```python
from build123d import *

# Parameters (mm, degrees)
SKETCH_1_W               = 124
SKETCH_1_H               = 43
EXTRUDE_1_DEPTH          = 1.2
CUT_EXTRUDE_1_REACH      = 110.402
SKETCH_3_W               = 7.4
SKETCH_3_H               = 4.6
SKETCH_3_W_2             = 4.6
CUT_EXTRUDE_2_DEPTH      = 0.4
FILLET_1_R               = 3
EXTRUDE_START            = 5
EXTRUDE_5_DEPTH          = 5
SKETCH_7_W               = 0.8
SKETCH_7_H               = 5.4
EXTRUDE_6_DEPTH          = 33.335489
SKETCH_8_W               = 4.5
SKETCH_8_H               = 0.8
CUT_EXTRUDE_3_DEPTH      = 5
CHAMFER_2_SIZE           = 0.5
CUT_EXTRUDE_5_DEPTH      = 109.510329697
CUT_EXTRUDE_5_DEPTH_BACK = 109.510329697
FILLET_2_R               = 3
FILLET_3_R               = 1
FILLET_4_R               = 0.5
SKETCH_10_W              = 10
SKETCH_10_H              = 0.8
CUT_EXTRUDE_6_DEPTH      = 5


with BuildPart() as part:
    # Эскиз1 → Бобышка-Вытянуть1 (new body)
    with BuildSketch(Plane(origin=(0, 0, 0), x_dir=(1, 0, 0), z_dir=(0, 1, 0))):
        with Locations((43.92682215, 1.5)):
            Rectangle(SKETCH_1_W, SKETCH_1_H)
    extrude(amount=EXTRUDE_1_DEPTH)

    # Эскиз3 → Вырез-Вытянуть1 (cut, up to next)
    with BuildSketch(Plane.XZ, mode=Mode.PRIVATE) as cut_extrude_1_sk1:
        with Locations((-7.87317785, -0.05)):
            Rectangle(SKETCH_3_W, SKETCH_3_H)
    cut_extrude_1_tool1 = extrude(cut_extrude_1_sk1.sketch, amount=-CUT_EXTRUDE_1_REACH, mode=Mode.PRIVATE) & part.part
    # Эскиз3 → Вырез-Вытянуть1 (cut, up to next)
    with BuildSketch(Plane.XZ, mode=Mode.PRIVATE) as cut_extrude_1_sk2:
        with Locations((-7.57317785, -7.75)):
            Rectangle(SKETCH_3_W_2, SKETCH_3_H)
    cut_extrude_1_tool2 = extrude(cut_extrude_1_sk2.sketch, amount=-CUT_EXTRUDE_1_REACH, mode=Mode.PRIVATE) & part.part
    add(cut_extrude_1_tool1.solids().sort_by_distance((-7.873178, 0, -0.05))[0], mode=Mode.SUBTRACT)
    add(cut_extrude_1_tool2.solids().sort_by_distance((-7.573178, 0, -7.75))[0], mode=Mode.SUBTRACT)

    # Эскиз4 → Вырез-Вытянуть2 (cut)
    with BuildSketch(Plane(origin=(0, 1.2, 0), x_dir=(1, 0, 0), z_dir=(0, 1, 0))):
        with BuildLine():
            Line((4.110011464, 20.25), (7.343632837, 20.25))
            Line((7.343632837, 20.25), (29.42682215, 20.25))
            Line((29.42682215, 20.25), (29.42682215, -13.75))
            ThreePointArc((29.42682215, -13.75), (28.401695885, -16.224873734), (25.92682215, -17.25))
            Line((25.92682215, -17.25), (-13.07317785, -17.25))
            ThreePointArc((-13.07317785, -17.25), (-15.548051584, -16.224873734), (-16.57317785, -13.75))
            Line((-16.57317785, -13.75), (-16.57317785, 16.75))
            ThreePointArc((-16.57317785, 16.75), (-15.548051584, 19.224873734), (-13.07317785, 20.25))
            Line((-13.07317785, 20.25), (4.110011464, 20.25))
        make_face()
    extrude(amount=-CUT_EXTRUDE_2_DEPTH, mode=Mode.SUBTRACT)

    # Скругление1
    fillet_1_edges = [part.edges().sort_by_distance(p)[0] for p in [
        (-18.07317785, 0.6, -23),
        (105.92682215, 0.6, -23),
        (105.92682215, 0.6, 20),
        (-18.07317785, 0.6, 20),
    ]]
    fillet(fillet_1_edges, radius=FILLET_1_R)

    # Эскиз5 → Бобышка-Вытянуть5 (add)
    with BuildSketch(Plane(origin=(0, 1.2, 0), x_dir=(1, 0, 0), z_dir=(0, 1, 0)).offset(EXTRUDE_START)):
        with BuildLine():
            ThreePointArc((102.92682215, -19), (104.341035713, -18.414213562), (104.92682215, -17))
            Line((104.92682215, -17), (104.92682215, 20))
            ThreePointArc((104.92682215, 20), (104.341035713, 21.414213562), (102.92682215, 22))
            Line((102.92682215, 22), (-15.07317785, 22))
            ThreePointArc((-15.07317785, 22), (-16.487391412, 21.414213562), (-17.07317785, 20))
            Line((-17.07317785, 20), (-17.07317785, -17))
            ThreePointArc((-17.07317785, -17), (-16.487391412, -18.414213562), (-15.07317785, -19))
            Line((-15.07317785, -19), (102.92682215, -19))
        make_face()
        with BuildLine():
            Line((102.92682215, -18.2), (-15.07317785, -18.2))
            ThreePointArc((-15.07317785, -18.2), (-15.921705987, -17.848528137), (-16.27317785, -17))
            Line((-16.27317785, -17), (-16.27317785, -15.167744688))
            ThreePointArc((-16.27317785, -15.167744688), (-16.497356583, -14.474568837), (-16.57317785, -13.75))
            Line((-16.57317785, -13.75), (-16.57317785, 16.75))
            ThreePointArc((-16.57317785, 16.75), (-16.497356583, 17.474568837), (-16.27317785, 18.167744688))
            Line((-16.27317785, 18.167744688), (-16.27317785, 20))
            ThreePointArc((-16.27317785, 20), (-15.921705987, 20.848528137), (-15.07317785, 21.2))
            Line((-15.07317785, 21.2), (102.92682215, 21.2))
            ThreePointArc((102.92682215, 21.2), (103.775350288, 20.848528137), (104.12682215, 20))
            Line((104.12682215, 20), (104.12682215, -17))
            ThreePointArc((104.12682215, -17), (103.775350288, -17.848528137), (102.92682215, -18.2))
        make_face(mode=Mode.SUBTRACT)
    extrude(amount=-EXTRUDE_5_DEPTH)

    # Эскиз7 → Бобышка-Вытянуть6 (add)
    with BuildSketch(Plane(origin=(0, 0, 15.167744688), x_dir=(-1, 0, 0), z_dir=(0, 0, -1))):
        with Locations((16.67317785, 3.5)):
            Rectangle(SKETCH_7_W, SKETCH_7_H)
    extrude(amount=EXTRUDE_6_DEPTH)

    # Эскиз8 → Вырез-Вытянуть3 (cut)
    with BuildSketch(Plane(origin=(0, 6.2, 0), x_dir=(1, 0, 0), z_dir=(0, 1, 0))):
        with Locations((7.97682215, 21.6)):
            Rectangle(SKETCH_8_W, SKETCH_8_H)
        with Locations((3.47682215, 21.6)):
            Rectangle(SKETCH_8_W, SKETCH_8_H)
    extrude(amount=-CUT_EXTRUDE_3_DEPTH, mode=Mode.SUBTRACT)

    # Фаска2
    chamfer_2_edges = [part.edges().sort_by_distance(p)[0] for p in [
        (1.22682215, 3.7, -22),
        (10.22682215, 3.7, -22),
    ]]
    chamfer(chamfer_2_edges, length=CHAMFER_2_SIZE)

    # Эскиз9 → Вырез-Вытянуть5 (cut, two sides: drawn at the far end of the back side and taken through both)
    with BuildSketch(Plane(origin=(0, 1.2, 0), x_dir=(1, 0, 0), z_dir=(0, 1, 0)).offset(-CUT_EXTRUDE_5_DEPTH_BACK)):
        Polygon((1.22682215, 21.5), (10.22682215, 21.5), (10.72682215, 22), (11.72682215, 23), (-0.27317785, 23), (0.72682215, 22), align=None)
    extrude(amount=CUT_EXTRUDE_5_DEPTH + CUT_EXTRUDE_5_DEPTH_BACK, mode=Mode.SUBTRACT)

    # Скругление2
    fillet_2_edges = [part.edges().sort_by_distance(p)[0] for p in [
        (-0.27317785, 0.6, -23),
        (11.72682215, 0.6, -23),
    ]]
    fillet(fillet_2_edges, radius=FILLET_2_R)

    # Скругление3
    fillet_3_edges = [part.edges().sort_by_distance(p)[0] for p in [
        (1.22682215, 0.6, -21.5),
        (10.22682215, 0.6, -21.5),
    ]]
    fillet(fillet_3_edges, radius=FILLET_3_R)

    # Скругление4
    # the kernel refuses this fillet: 0.5 mm, written as the material it takes off along each edge
    with BuildSketch(Plane(origin=(9.812608588, 1.2, -21.5), x_dir=(0, 0, 1), z_dir=(-1, 0, 0))) as fillet_4_piece_1:
        with BuildLine():
            CenterArc((FILLET_4_R, -FILLET_4_R), FILLET_4_R, 90, 90)
            Line((0, -FILLET_4_R), (0, 0))
            Line((0, 0), (FILLET_4_R, 0))
        make_face()
    extrude(amount=8.171572875, mode=Mode.SUBTRACT)
    with BuildSketch(Plane(origin=(1.641035713, 1.2, -22.5), x_dir=(-0.8939437975787546, 0, -0.448179078907611), z_dir=(0.448179078907611, 0, -0.8939437975787546))) as fillet_4_piece_2_section:
        with BuildLine():
            CenterArc((1 + FILLET_4_R, -FILLET_4_R), FILLET_4_R, 90, 90)
            Line((1, -FILLET_4_R), (1, 0))
            Line((1, 0), (1 + FILLET_4_R, 0))
        make_face()
    fillet_4_piece_2 = revolve(axis=Axis((1.641035713, 1.2, -22.5), (0, 1, 0)), revolution_arc=116.626915432, mode=Mode.PRIVATE)
    fillet_4_piece_2 = split(fillet_4_piece_2, bisect_by=Plane(origin=(1.130412309, 1.014643197, -21.596409841), z_dir=(0.7071067811865498, 0, -0.7071067811865454)), keep=Keep.TOP, mode=Mode.PRIVATE)
    add(fillet_4_piece_2, mode=Mode.SUBTRACT)
    with BuildSketch(Plane(origin=(1.641035713, 1.2, -22.5), x_dir=(-0.8939437975787546, 0, -0.448179078907611), z_dir=(0.448179078907611, 0, -0.8939437975787546))) as fillet_4_piece_3_section:
        with BuildLine():
            CenterArc((1 + FILLET_4_R, -FILLET_4_R), FILLET_4_R, 90, 90)
            Line((1, -FILLET_4_R), (1, 0))
            Line((1, 0), (1 + FILLET_4_R, 0))
        make_face()
    fillet_4_piece_3 = revolve(axis=Axis((1.641035713, 1.2, -22.5), (0, 1, 0)), revolution_arc=116.626915432, mode=Mode.PRIVATE)
    fillet_4_piece_3 = split(fillet_4_piece_3, bisect_by=Plane(origin=(1.22682215, 1.150324025, -21.336464166), z_dir=(1, 0, 0)), keep=Keep.TOP, mode=Mode.PRIVATE)
    add(fillet_4_piece_3, mode=Mode.SUBTRACT)
    with BuildSketch(Plane(origin=(1.641035713, 1.2, -22.5), x_dir=(-0.8939437975787546, 0, -0.448179078907611), z_dir=(0.448179078907611, 0, -0.8939437975787546))) as fillet_4_piece_4_section:
        with BuildLine():
            CenterArc((1 + FILLET_4_R, -FILLET_4_R), FILLET_4_R, 90, 90)
            Line((1, -FILLET_4_R), (1, 0))
            Line((1, 0), (1 + FILLET_4_R, 0))
        make_face()
    fillet_4_piece_4 = revolve(axis=Axis((1.641035713, 1.2, -22.5), (0, 1, 0)), revolution_arc=116.626915432, mode=Mode.PRIVATE)
    fillet_4_piece_4 = split(fillet_4_piece_4, bisect_by=Plane(origin=(1.152970199, 1.196161592, -21.2), z_dir=(0, 0, 1)), keep=Keep.TOP, mode=Mode.PRIVATE)
    add(fillet_4_piece_4, mode=Mode.SUBTRACT)
    with BuildSketch(Plane(origin=(9.812608588, 1.2, -22.5), x_dir=(0.8939437975787601, 0, -0.4481790789075999), z_dir=(-0.4481790789075999, 0, -0.8939437975787601))) as fillet_4_piece_5_section:
        with BuildLine():
            CenterArc((1 + FILLET_4_R, FILLET_4_R), FILLET_4_R, 180, 90)
            Line((1 + FILLET_4_R, 0), (1, 0))
            Line((1, 0), (1, FILLET_4_R))
        make_face()
    fillet_4_piece_5 = revolve(axis=Axis((9.812608588, 1.2, -22.5), (0, -1, 0)), revolution_arc=116.626915432, mode=Mode.PRIVATE)
    fillet_4_piece_5 = split(fillet_4_piece_5, bisect_by=Plane(origin=(10.323231991, 1.014642922, -21.59640984), z_dir=(-0.7071067811865426, 0, -0.7071067811865526)), keep=Keep.TOP, mode=Mode.PRIVATE)
    add(fillet_4_piece_5, mode=Mode.SUBTRACT)
    with BuildSketch(Plane(origin=(9.812608588, 1.2, -22.5), x_dir=(0.8939437975787601, 0, -0.4481790789075999), z_dir=(-0.4481790789075999, 0, -0.8939437975787601))) as fillet_4_piece_6_section:
        with BuildLine():
            CenterArc((1 + FILLET_4_R, FILLET_4_R), FILLET_4_R, 180, 90)
            Line((1 + FILLET_4_R, 0), (1, 0))
            Line((1, 0), (1, FILLET_4_R))
        make_face()
    fillet_4_piece_6 = revolve(axis=Axis((9.812608588, 1.2, -22.5), (0, -1, 0)), revolution_arc=116.626915432, mode=Mode.PRIVATE)
    fillet_4_piece_6 = split(fillet_4_piece_6, bisect_by=Plane(origin=(10.22682215, 1.150324024, -21.336464168), z_dir=(-1, 0, 0)), keep=Keep.TOP, mode=Mode.PRIVATE)
    add(fillet_4_piece_6, mode=Mode.SUBTRACT)
    with BuildSketch(Plane(origin=(9.812608588, 1.2, -22.5), x_dir=(0.8939437975787601, 0, -0.4481790789075999), z_dir=(-0.4481790789075999, 0, -0.8939437975787601))) as fillet_4_piece_7_section:
        with BuildLine():
            CenterArc((1 + FILLET_4_R, FILLET_4_R), FILLET_4_R, 180, 90)
            Line((1 + FILLET_4_R, 0), (1, 0))
            Line((1, 0), (1, FILLET_4_R))
        make_face()
    fillet_4_piece_7 = revolve(axis=Axis((9.812608588, 1.2, -22.5), (0, -1, 0)), revolution_arc=116.626915432, mode=Mode.PRIVATE)
    fillet_4_piece_7 = split(fillet_4_piece_7, bisect_by=Plane(origin=(10.300674101, 1.196161592, -21.2), z_dir=(0, 0, 1)), keep=Keep.TOP, mode=Mode.PRIVATE)
    add(fillet_4_piece_7, mode=Mode.SUBTRACT)

    # Эскиз10 → Вырез-Вытянуть6 (cut)
    with BuildSketch(Plane(origin=(0, 6.2, 0), x_dir=(1, 0, 0), z_dir=(0, 1, 0))):
        with Locations((-8.57317785, -18.6)):
            Rectangle(SKETCH_10_W, SKETCH_10_H)
    extrude(amount=-CUT_EXTRUDE_6_DEPTH, mode=Mode.SUBTRACT)


solid = part.part
```
Check sheet for the modelled part. Datum: model origin and axes. Units: mm. A direction names the side the tool comes from. Round coordinates to 2 decimals unless told otherwise and drop trailing zeros. Loops run counter-clockwise (first coordinate to the right, second up) from the corner with the lowest first, then second, coordinate; pieces in that order, holes last. Notation, with made-up numbers: (10, -13) -> (16, -13) arc R16 cw to (16, -2) -> close; hole circle Ø8 at (3, 68). An arc over 180 degrees is marked (long way). Write item = value, one per line. Start each with the question number.
1) Sectioned sample at C-C, the plane y = 3. Record the cut outline in (x, z).
2) Thickness scan on probe 1 along Z at (x, y) = (87, 1.25); probe 2 along X at (y, z) = (5.5, 2); probe 3 along Y at (x, z) = (10, 6.5). Record the ranges inside material, lowest first.
3) Set-up check for faces 1 (the flat face through (49, 4, 19)), 2 (the flat face through (104.127, 4, -2)), 3 (the flat face through (-17.073, 4, -2)), 4 (the flat face through (57, 4, -22)): record each of +Z, -Z, +X, -X, +Y, -Y from which the full face is reachable in a straight line by a thin tool's end or side.
4) Sectioned sample at B-B, the plane x = 22. Record the cut outline in (y, z), plus the area to 3 significant figures.
5) Sectioned sample at D-D, the plane x = 86. Record the cut outline in (y, z), plus the area to 3 significant figures.
6) Gauge pin test, flat ends, axial feed: pin 1 Ø1.5 at (y, z) = (2.5, 2.5) entering from -X; pin 2 Ø3 at (y, z) = (4, 9.5) entering from +X. Record the tip position at first contact, or that the pin passes through.
7) Release check for a two-part mould opening along Z. For faces 5 (the flat face through (50, 4, 18.2)), 6 (the cylindrical face through (-16.5, 3.7, -21.4)), 7 (the cylindrical face through (105.025, 0.608, 19.145)) record: released by +Z, released by -Z, zero draft, split by the parting line, or undercut.
8) Sectioned sample at A-A, the plane z = 0.5. Record the cut outline in (x, y).
Results are:
q1.outline = (-17.07, -20) arc R2 ccw to (-15.07, -22) -> (0.73, -22) -> (1.23, -21.5) -> (1.23, -21.2) -> (-15.07, -21.2) arc R1.2 cw to (-16.27, -20) -> (-16.27, 17) arc R1.2 cw to (-15.07, 18.2) -> (-13.57, 18.2) -> (-13.57, 19) -> (-15.07, 19) arc R2 ccw to (-17.07, 17) -> close; (-3.57, 18.2) -> (102.93, 18.2) arc R1.2 cw to (104.13, 17) -> (104.13, -20) arc R1.2 cw to (102.93, -21.2) -> (10.23, -21.2) -> (10.23, -21.5) -> (10.73, -22) -> (102.93, -22) arc R2 ccw to (104.93, -20) -> (104.93, 17) arc R2 ccw to (102.93, 19) -> (-3.57, 19) -> close
q2.probe_1 = -22 to -21.2, 18.2 to 19
q2.probe_2 = -17.07 to -16.27, 104.13 to 104.93
q2.probe_3 = 0 to 0.8
q3.face_1 = +Z, +X, -X, +Y
q3.face_2 = +Y
q3.face_3 = +Z, -Z, -X, +Y
q3.face_4 = -Z, +X, -X, +Y
q4.outline = (0, -23) -> (1.2, -23) -> (1.2, -22) -> (6.2, -22) -> (6.2, -21.2) -> (1.2, -21.2) -> (1.2, -20.25) -> (0.8, -20.25) -> (0.8, 17.25) -> (1.2, 17.25) -> (1.2, 18.2) -> (6.2, 18.2) -> (6.2, 19) -> (1.2, 19) -> (1.2, 20) -> (0, 20) -> close
q4.area = 44.6 mm^2
q5.outline = (0, -23) -> (1.2, -23) -> (1.2, -22) -> (6.2, -22) -> (6.2, -21.2) -> (1.2, -21.2) -> (1.2, 18.2) -> (6.2, 18.2) -> (6.2, 19) -> (1.2, 19) -> (1.2, 20) -> (0, 20) -> close
q5.area = 59.6 mm^2
q6.pin_1 = -17.07
q6.pin_2 = 104.93
q7.face_5 = undercut
q7.face_6 = released by -Z
q7.face_7 = released by +Z
q8.outline = (-18.07, 0) -> (-11.57, 0) -> (-11.57, 0.8) -> (-16.27, 0.8) -> (-16.27, 6.2) -> (-17.07, 6.2) -> (-17.07, 1.2) -> (-18.07, 1.2) -> close; (-4.17, 0) -> (105.93, 0) -> (105.93, 1.2) -> (104.93, 1.2) -> (104.93, 6.2) -> (104.13, 6.2) -> (104.13, 1.2) -> (29.43, 1.2) -> (29.43, 0.8) -> (-4.17, 0.8) -> close
